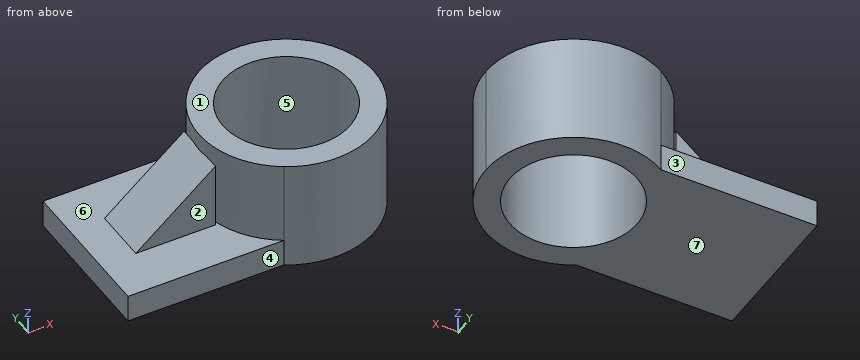
from build123d import *

# Parameters (mm, degrees)
F1_DEPTH = 12.7
F0_R     = 29.196285
F2_DEPTH = 50.8
F4_DEPTH = 12.7


with BuildPart() as f1:
    # F0 (on Top) → F1 (new body)
    with BuildSketch(Plane.XY):
        with BuildLine():
            Line((25.401515, 34.4395), (-46.141323, 34.4395))
            Line((-46.141323, 34.4395), (-46.141323, -34.4395))
            Line((-46.141323, -34.4395), (25.401515, -34.4395))
            ThreePointArc((25.401515, -34.4395), (5.939099, 0), (25.401515, 34.4395))
        make_face()
    extrude(amount=F1_DEPTH)

    # F0 (on Top) → F2 (join)
    with BuildSketch(Plane.XY):
        with BuildLine():
            ThreePointArc((86.343547, 0), (65.920509, 35.000037), (25.401515, 34.4395))
            ThreePointArc((25.401515, 34.4395), (5.939099, 0), (25.401515, -34.4395))
            ThreePointArc((25.401515, -34.4395), (65.920509, -35.000037), (86.343547, 0))
        make_face()
        with Locations((46.141323, 0)):
            Circle(F0_R, mode=Mode.SUBTRACT)
    extrude(amount=F2_DEPTH)

    # F3 (on Front) → F4 (join, symmetric)
    with BuildSketch(Plane.XZ):
        Polygon((6.308553, 12.938597), (6.308553, 43.192081), (-30.223956, 12.938597), align=None)
    extrude(amount=F4_DEPTH, both=True)


solid = f1.part
Source: CAD feature listing. Evaluate the final solid. Frame: model axes, mm. Face numbers are marked on the shaded views. A direction names the side the tool comes from. Round coordinates to 2 decimals unless told otherwise and drop trailing zeros. Loops run counter-clockwise (first coordinate to the right, second up) from the corner with the lowest first, then second, coordinate; pieces in that order, holes last. Notation, with made-up numbers: M 27,27 L 43,27 A20 cw 43,31 Z; hole C -24,49.25 d6. An arc over 180 degrees is marked long. Return JSON: item names as keys, results as strings. Group by question number.
1. Reachability of the marked faces 1, 2, 3 and 4 from +Z, -Z, +X, -X, +Y, -Y: full face, straight path, thin tool, end or side. Return the list, or none.
2. Section query C-C on z = 15. Output: boundary loops of the cut face in (x, y).
3. Mould query, pull axis Z, two halves, no side actions, for the marked faces 5, 6 and 7. Classes: released by +Z, released by -Z, zero draft, split by the parting line, or undercut.
4. Section query B-B on y = -15. Output: boundary loops of the cut face in (x, z).
5. Pin query (flat end, axial travel): pin 1 (10 mm diameter, centred on x = -23, z = 8.5, fed in from +Y); pin 2 (8 mm diameter, centred on y = -7.5, z = 21, fed in from +X); pin 3 (12 mm diameter, centred on x = 68, z = 19.5, fed in from +Y); pin 4 (9 mm diameter, centred on x = -18.5, z = 31, fed in from -Y). Return the tip coordinate at first contact, or that it passes through.
6. Section query A-A on x = 54. Output: boundary loops of the cut face in (y, z), and give its area (3 significant figures).
7. Section query D-D on z = 25.5. Output: boundary loops of the cut face in (x, y), and give its area (3 significant figures).
8. Material intervals for line 1 along Y through (x, z) = (-25.5, 6); line 2 along Y through (x, z) = (-2, 15); line 3 along X through (y, z) = (-24, 16.5), sorted ascending. Write a range as from..to.
Checks:
{
 "1": {"face 1": "+Z, +X, -X, +Y, -Y", "face 2": "+Z, -X, -Y", "face 3": "+Z, -Z, -X, +Y", "face 4": "+Z, -Z, -X, -Y"},
 "2": {"outline": "M -27.73,-12.7 L 6.31,-12.7 L 6.31,-5.44 A40.2 ccw long 6.31,5.44 L 6.31,12.7 L -27.73,12.7 Z; hole C 46.14,0 d58.39"},
 "3": {"face 5": "zero draft", "face 6": "undercut", "face 7": "released by -Z"},
 "4": {"outline": "M -46.14,0 L 21.09,0 L 21.09,50.8 L 8.84,50.8 L 8.84,12.7 L -46.14,12.7 Z; M 71.19,0 L 83.44,0 L 83.44,50.8 L 71.19,50.8 Z"},
 "5": {"pin 1": "stops at y = 34.44", "pin 2": "stops at x = 86.19", "pin 3": "stops at y = 36.94", "pin 4": "passes through"},
 "6": {"outline": "M -39.43,0 L -28.12,0 L -28.12,50.8 L -39.43,50.8 Z; M 28.12,0 L 39.43,0 L 39.43,50.8 L 28.12,50.8 Z", "area": "1,150 mm²"},
 "7": {"outline": "M -15.06,-12.7 L 6.31,-12.7 L 6.31,-5.44 A40.2 ccw long 6.31,5.44 L 6.31,12.7 L -15.06,12.7 Z; hole C 46.14,0 d58.39", "area": "2,940 mm²"},
 "8": {"line 1": "y = -34.44..34.44", "line 2": "y = -12.7..12.7", "line 3": "x = 13.89..29.52, 62.77..78.39"}
}
